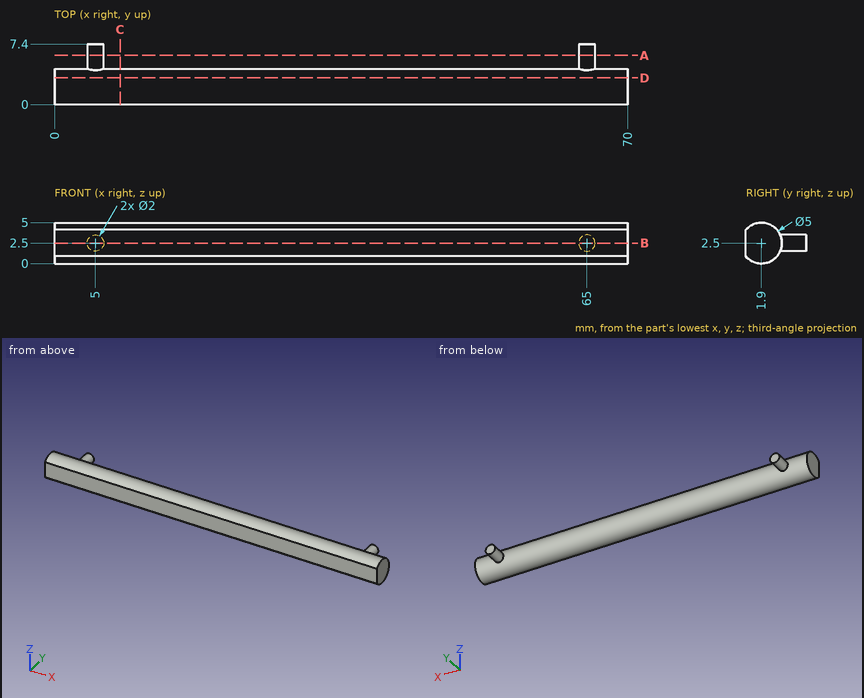
Source: three-view drawing plus pictorial views. Frame: mm from the lowest corner of the part. Give positions to 0.01 mm unless a question says otherwise; leave off trailing zeros. Loops run counter-clockwise (first coordinate to the right, second up) from the corner with the lowest first, then second, coordinate; pieces in that order, holes last. Notation, with made-up numbers: (18.25, 7) -> (43.25, 7) arc R11 cw to (43.25, 25) -> close; hole circle Ø4 at (-18, 9). An arc over 180 degrees is marked (long way). Put each result on its own line as item: value. Start each with the question number.
1) Material intervals for probe 1 along Y at (x, z) = (64, 3.5); probe 2 along X at (y, z) = (6.5, 1.9); probe 3 along X at (y, z) = (7, 3), sorted ascending.
2) Cut plane D-D (y = 3.25). Return loops of the section in (x, z).
3) Cut plane C-C (x = 8). Return loops of the section in (y, z).
4) Cut plane A-A (y = 6). Return loops of the section in (x, z).
5) Cut plane B-B (z = 2.5). Return loops of the section in (x, y).
6) Contact query for flat-ended pins moving along their axis: P1, Ø1.5, axis at x = 35, y = 4.5, coming from the -Z side; P2, Ø3, axis at x = 30, y = 6, coming from the -Z side; P3, Ø4, axis at x = 31, y = 5, coming from the -Z side (3 decimals); P4, Ø1, axis at y = 4, z = 4, coming from the -X side. Output: stop coordinate, or through.
Results are:
1. probe 1: y = 0 to 4.19
1. probe 2: x = 4.2 to 5.8, 64.2 to 65.8
1. probe 3: x = 4.13 to 5.87, 64.13 to 65.87
2. outline: (0, 0.4) -> (70, 0.4) -> (70, 4.6) -> (0, 4.6) -> close
3. outline: (0, 0.88) arc R2.5 ccw (long way) to (0, 4.12) -> close
4. outline: circle Ø2 at (5, 2.5); circle Ø2 at (65, 2.5)
5. outline: (0, 0) -> (70, 0) -> (70, 4.4) -> (66, 4.4) -> (66, 7.4) -> (64, 7.4) -> (64, 4.4) -> (6, 4.4) -> (6, 7.4) -> (4, 7.4) -> (4, 4.4) -> (0, 4.4) -> close
6. P1: stops at z = 0.82
6. P2: passes through
6. P3: stops at z = 0.255
6. P4: stops at x = 0
